```python
from build123d import *

# Parameters (mm, degrees)
SKETCH1_W           = 90
SKETCH1_H           = 125
BOSS_EXTRUDE1_DEPTH = 12
SKETCH2_W           = 12.5
SKETCH2_H           = 125
BOSS_EXTRUDE2_DEPTH = 22
SKETCH3_W           = 38.75
SKETCH3_H           = 89
SKETCH3_W_2         = 6.25
BOSS_EXTRUDE3_DEPTH = 12
SKETCH4_W           = 92.043364018
SKETCH4_H           = 5.697421696
CUT_EXTRUDE1_DEPTH  = 143.714969432


with BuildPart() as part:
    # Sketch1 → Boss-Extrude1 (new body)
    with BuildSketch(Plane(origin=(0, 0, 0), x_dir=(1, 0, 0), z_dir=(0, 1, 0))):
        with Locations((45, 62.5)):
            Rectangle(SKETCH1_W, SKETCH1_H)
    extrude(amount=BOSS_EXTRUDE1_DEPTH)

    # Sketch2 → Boss-Extrude2 (add)
    with BuildSketch(Plane(origin=(0, 12, 0), x_dir=(1, 0, 0), z_dir=(0, 1, 0))):
        with Locations((45, 62.5)):
            Rectangle(SKETCH2_W, SKETCH2_H)
    extrude(amount=BOSS_EXTRUDE2_DEPTH)

    # Sketch3 → Boss-Extrude3 (add)
    with BuildSketch(Plane(origin=(0, 34, 0), x_dir=(1, 0, 0), z_dir=(0, 1, 0))):
        with Locations((70.625, 80.5)):
            Rectangle(SKETCH3_W, SKETCH3_H)
        with Locations((19.375, 80.5)):
            Rectangle(SKETCH3_W, SKETCH3_H)
        with Locations((41.875, 80.5)):
            Rectangle(SKETCH3_W_2, SKETCH3_H)
        with Locations((48.125, 80.5)):
            Rectangle(SKETCH3_W_2, SKETCH3_H)
    extrude(amount=BOSS_EXTRUDE3_DEPTH)

    # Sketch4 → Cut-Extrude1 (cut, through all)
    with BuildSketch(Plane(origin=(51.25, 0, 0), x_dir=(0, 0, -1), z_dir=(1, 0, 0))):
        with Locations((78.978317991, 14.848710848)):
            Rectangle(SKETCH4_W, SKETCH4_H)
    extrude(amount=-CUT_EXTRUDE1_DEPTH, mode=Mode.SUBTRACT)


solid = part.part
```
The listing builds one solid part. Answer for the finished solid, in the listing's coordinates (mm). A direction names the side the tool comes from. Coordinates: 2 decimals unless noted, no trailing zeros. Write each loop counter-clockwise with the first axis right and the second up, starting at its lowest first coordinate (ties: lowest second). Pieces come first, ordered by that corner, then holes. Notation, with made-up numbers: (26, 71) - (45, 71) arc R21 cw to (45, 84) - close; hole circle Ø9 at (-11.5, -3.75). An arc over 180 degrees is marked (long way). Return JSON: item names as keys, results as strings. Group by question number.
1. A cutting plane is placed at C-C, the plane x = 45. Determine the outline of the cut face in (y, z), plus the area to 3 significant figures.
2. Given pin 1 (6 mm diameter, centred on x = 35.5, y = 34.5, fed in from +Z); pin 2 (6.5 mm diameter, centred on y = 22, z = -78.5, fed in from -X); pin 3 (1.7 mm diameter, centred on x = 42, y = 14, fed in from -Z), each flat-ended and moving along its own axis, determine where each tip first touches the part or whether it passes through.
3. Straight lines are drawn through the part: L1, parallel to Y at x = 63, z = -104.5; L2, parallel to Y at x = 39, z = -46.5; L3, parallel to Y at x = 23.5, z = -17. For each, find the intervals that lie inside material, in ascending order.
4. A cutting plane is placed at B-B, the plane x = 76. Determine the outline of the cut face in (y, z).
5. A cutting plane is placed at D-D, the plane z = -34.5. Determine the outline of the cut face in (x, y), plus the area to 3 significant figures.
6. A cutting plane is placed at A-A, the plane z = -90. Determine the outline of the cut face in (x, y).
7. Determine the mould class of faces 4 (the flat face through (38.75, 25, -62)), 5 (the flat face through (44, 9, 0)), 6 (the flat face through (44, 0, -63)) for opening direction Y: released by +Y, released by -Y, zero draft, split by the parting line, or undercut.
8. Which of the six approach directions +Z, -Z, +X, -X, +Y, -Y give full straight-line access (tool end or side, diameter ignored) to faces 1 (the flat face through (45, 15, -32.957)), 2 (the flat face through (44, 40, -36)), 3 (the flat face through (51.25, 25, -62))?
Ans:
{
 "1": {"outline": "(0, -125) - (12, -125) - (12, -32.96) - (17.7, -32.96) - (17.7, -125) - (46, -125) - (46, -36) - (34, -36) - (34, 0) - (0, 0) - close", "area": "4,790 mm²"},
 "2": {"pin 1": "z = -36", "pin 2": "x = 38.75", "pin 3": "z = -32.96"},
 "3": {"L1": "0 to 12, 34 to 46", "L2": "0 to 12, 17.7 to 46", "L3": "0 to 12"},
 "4": {"outline": "(0, -125) - (12, -125) - (12, 0) - (0, 0) - close; (34, -125) - (46, -125) - (46, -36) - (34, -36) - close"},
 "5": {"outline": "(0, 0) - (90, 0) - (90, 12) - (0, 12) - close; (38.75, 17.7) - (51.25, 17.7) - (51.25, 34) - (38.75, 34) - close", "area": "1,280 mm²"},
 "6": {"outline": "(0, 0) - (90, 0) - (90, 12) - (0, 12) - close; (0, 34) - (38.75, 34) - (38.75, 17.7) - (51.25, 17.7) - (51.25, 34) - (90, 34) - (90, 46) - (0, 46) - close"},
 "7": {"face 4": "undercut", "face 5": "zero draft", "face 6": "released by -Y"},
 "8": {"face 1": "-Z, +X, -X", "face 2": "+Z, +X, -X, +Y", "face 3": "+Z, -Z, +X"}
}
